Can you work these out from the model? Positions are in its coordinate system, mm. A direction names the side the tool comes from. Round coordinates to 2 decimals unless told otherwise and drop trailing zeros. Loops run counter-clockwise (first coordinate to the right, second up) from the corner with the lowest first, then second, coordinate; pieces in that order, holes last. Notation, with made-up numbers: M 86,34 L 126,34 A16 cw 126,58 Z; hole C 75.5,76 d9. An arc over 180 degrees is marked long. Return JSON: item names as keys, results as strings.
```python
from build123d import *
from OCP.BRepFilletAPI import BRepFilletAPI_MakeChamfer

# Parameters (mm, degrees)
SKETCH1_W           = 42
SKETCH1_H           = 42
SKETCH1_R           = 12
SKETCH1_R_2         = 1.5
BOSS_EXTRUDE1_DEPTH = 6
CHAMFER1_SIZE       = 2
SKETCH2_W           = 24
SKETCH2_H           = 21
CUT_EXTRUDE1_DEPTH  = 31.298514815
CHAMFER2_SIZE       = 4.5
CHAMFER2_SIZE2      = 1.205771366


with BuildPart() as part:
    # Sketch1 → Boss-Extrude1 (new body)
    with BuildSketch(Plane(origin=(0, 0, 0), x_dir=(1, 0, 0), z_dir=(0, 1, 0))):
        Rectangle(SKETCH1_W, SKETCH1_H)
        with Locations(Location((0, 0, 0), (0, 0, 270))):
            Circle(SKETCH1_R, mode=Mode.SUBTRACT)
        with Locations(Location((-15.5, 15.5, 0), (0, 0, 270))):
            Circle(SKETCH1_R_2, mode=Mode.SUBTRACT)
        with Locations(Location((15.5, 15.5, 0), (0, 0, 270))):
            Circle(SKETCH1_R_2, mode=Mode.SUBTRACT)
        with Locations(Location((15.5, -15.5, 0), (0, 0, 270))):
            Circle(SKETCH1_R_2, mode=Mode.SUBTRACT)
        with Locations(Location((-15.5, -15.5, 0), (0, 0, 270))):
            Circle(SKETCH1_R_2, mode=Mode.SUBTRACT)
    extrude(amount=BOSS_EXTRUDE1_DEPTH)

    # Chamfer1
    chamfer1_edges = [part.edges().sort_by_distance(p)[0] for p in [
        (21, 3, 21),
        (-21, 3, 21),
        (-21, 3, -21),
        (21, 3, -21),
    ]]
    chamfer(chamfer1_edges, length=CHAMFER1_SIZE)

    # Sketch2 → Cut-Extrude1 (cut, through all)
    with BuildSketch(Plane(origin=(0, 6, 0), x_dir=(1, 0, 0), z_dir=(0, 1, 0))):
        with Locations((0, -10.5)):
            Rectangle(SKETCH2_W, SKETCH2_H)
    extrude(amount=-CUT_EXTRUDE1_DEPTH, mode=Mode.SUBTRACT)

    # Chamfer2: one chamfer whose edges measure the first distance from different faces: ONE call of the kernel's chamfer builder (chamfer() names one face for all edges)
    chamfer2_edges_1 = [part.edges().sort_by_distance(p)[0] for p in [
        (12, 3, 21),
    ]]
    chamfer2_side_1 = [part.faces().sort_by_distance(p)[0] for p in [
        (12, 3, 10.5),
    ]]
    chamfer2_edges_2 = [part.edges().sort_by_distance(p)[0] for p in [
        (-12, 3, 21),
    ]]
    chamfer2_side_2 = [part.faces().sort_by_distance(p)[0] for p in [
        (-12, 3, 10.5),
    ]]
    chamfer2 = BRepFilletAPI_MakeChamfer(part.part.solid().wrapped)
    for e in chamfer2_edges_1:
        chamfer2.Add(CHAMFER2_SIZE, CHAMFER2_SIZE2, e.wrapped, chamfer2_side_1[0].wrapped)  # the first distance lies on this face
    for e in chamfer2_edges_2:
        chamfer2.Add(CHAMFER2_SIZE, CHAMFER2_SIZE2, e.wrapped, chamfer2_side_2[0].wrapped)  # the first distance lies on this face
    add(Compound.cast(chamfer2.Shape()), mode=Mode.REPLACE)


solid = part.part
```
Q1. If I drill on line 1 along X through (y, z) = (3.65, -15.5); line 2 along X through (y, z) = (4.1, 15.5); line 3 along X through (y, z) = (1.9, 3), over which ranges is the centre line in solid material (lowest first)?
Results:
{"line 1": "x = -21 to -17, -14 to 14, 17 to 21", "line 2": "x = -21 to -17, -14 to -12, 12 to 14, 17 to 21", "line 3": "x = -21 to -12, 12 to 21"}
Q2. Suppose I cut it at A-A, the plane z = -15.5. Please give me the cut outline in (x, y), plus the area to 3 significant figures.
Results:
{"outline": "M -21,0 L -17,0 L -17,6 L -21,6 Z; M -14,0 L 14,0 L 14,6 L -14,6 Z; M 17,0 L 21,0 L 21,6 L 17,6 Z", "area": "216 mm2"}
Q3. Suppose I cut it at B-B, the plane y = 4.8. Please give me the cut outline in (x, z).
Results:
{"outline": "M -21,-19 L -19,-21 L 19,-21 L 21,-19 L 21,19 L 19,21 L 13.21,21 L 12,16.5 L 12,0 A12 cw -12,0 L -12,16.5 L -13.21,21 L -19,21 L -21,19 Z; hole C -15.5,-15.5 d3; hole C -15.5,15.5 d3; hole C 15.5,-15.5 d3; hole C 15.5,15.5 d3"}
Q4. On a 3-axis mill with a long thin cutter (end or side, diameter ignored), from which of +Z, -Z, +X, -X, +Y, -Y can I reach the whole of each face in a straight line? I mean faces 4 (the flat face through (12, 3, 8)), 5 (the flat face through (-21, 3, 0)). Say none if no direction works.
Results:
{"face 4": "+Z, +Y, -Y", "face 5": "+Z, -Z, -X, +Y, -Y"}
Q5. Suppose I cut it at C-C, the plane x = -15.5. Please give me the cut outline in (y, z).
Results:
{"outline": "M 0,-21 L 6,-21 L 6,-17 L 0,-17 Z; M 0,-14 L 6,-14 L 6,14 L 0,14 Z; M 0,17 L 6,17 L 6,21 L 0,21 Z"}
Q6. Thinking about a two-plate mould opening in Z: for faces 1 (the flat face through (0, 0, -14)), 2 (the cylindrical face through (15.57, 2.96, -17)), 3 (the flat face through (16, 3, 21)), which applies, pulls with the +Z half, pulls with the -Z half, needs draft (parallel to the pull), parting line crosses it, or undercut?
Results:
{"face 1": "needs draft", "face 2": "undercut", "face 3": "pulls with the +Z half"}
Q7. I'm going to push a flat-ended pin straight in: pin 1 Ø1.8 at (x, z) = (15.5, 15.5) entering from +Y. Where does the tip first touch, or does it pass through?
Results:
{"pin 1": "passes through"}
Q8. Suppose I cut it at D-D, the plane z = 15.5. Please give me the cut outline in (x, y).
Results:
{"outline": "M -21,0 L -17,0 L -17,6 L -21,6 Z; M -14,0 L -12,0 L -12,6 L -14,6 Z; M 12,0 L 14,0 L 14,6 L 12,6 Z; M 17,0 L 21,0 L 21,6 L 17,6 Z"}
